```python
from build123d import *

# Parameters (mm, degrees)
SKETCH1_R               = 18
SKETCH1_R_2             = 16
BOSS_EXTRUDE1_DEPTH     = 50
SKETCH3_R               = 18
BOSS_EXTRUDE2_DEPTH     = 2
BOSS_EXTRUDE3_START     = -48
SKETCH3_2_R             = 18
BOSS_EXTRUDE3_DEPTH     = 2
CUT_EXTRUDE1_START      = 14
SKETCH2_W               = 50
SKETCH2_H               = 36
CUT_EXTRUDE1_DEPTH      = 150
CUT_EXTRUDE2_DEPTH      = 57.107040556
CUT_EXTRUDE2_DEPTH_BACK = 57.107040556
SKETCH4_R               = 4


with BuildPart() as part:
    # Sketch1 → Boss-Extrude1 (new body)
    with BuildSketch(Plane.XY):
        Circle(SKETCH1_R)
        Circle(SKETCH1_R_2, mode=Mode.SUBTRACT)
    extrude(amount=BOSS_EXTRUDE1_DEPTH)

    # Sketch3 → Boss-Extrude2 (add)
    with BuildSketch(Plane(origin=(0, 0, 0), x_dir=(-1, 0, 0), z_dir=(0, 0, -1))):
        with Locations(Location((0, 0, 0), (0, 0, 180))):
            Circle(SKETCH3_R)
    extrude(amount=-BOSS_EXTRUDE2_DEPTH)

    # Sketch3<2> → Boss-Extrude3 (add)
    with BuildSketch(Plane(origin=(0, 0, 0), x_dir=(-1, 0, 0), z_dir=(0, 0, -1)).offset(BOSS_EXTRUDE3_START)):
        with Locations(Location((0, 0, 0), (0, 0, 180))):
            Circle(SKETCH3_2_R)
    extrude(amount=-BOSS_EXTRUDE3_DEPTH)

    # Sketch2 → Cut-Extrude1 (cut)
    with BuildSketch(Plane(origin=(0, 0, 0), x_dir=(0, 0, -1), z_dir=(1, 0, 0)).offset(CUT_EXTRUDE1_START)):
        with Locations((-25, 0)):
            Rectangle(SKETCH2_W, SKETCH2_H)
    extrude(amount=CUT_EXTRUDE1_DEPTH, mode=Mode.SUBTRACT)

    # Sketch4 → Cut-Extrude2 (cut, two sides: drawn at the far end of the back side and taken through both)
    with BuildSketch(Plane.XY.offset(50).offset(-CUT_EXTRUDE2_DEPTH_BACK)):
        Circle(SKETCH4_R)
    extrude(amount=CUT_EXTRUDE2_DEPTH + CUT_EXTRUDE2_DEPTH_BACK, mode=Mode.SUBTRACT)


solid = part.part
```
For this review, take the finished solid that the model builds, in its own axes (mm). A direction names the side the tool comes from. Coordinates: 2 decimals unless noted, no trailing zeros. Write each loop counter-clockwise with the first axis right and the second up, starting at its lowest first coordinate (ties: lowest second). Pieces come first, ordered by that corner, then holes. Notation, with made-up numbers: (-18.5, 28) -> (26.5, 28) arc R14 cw to (26.5, 50) -> close; hole circle Ø1 at (18.25, 20). An arc over 180 degrees is marked (long way). Put each result on its own line as item: value.
Q1. Tool access review of faces 4 (the cylindrical face through (-0.867, -3.905, 48.986)), 5 (the flat face through (-5, 0, 2)): name each direction out of +Z, -Z, +X, -X, +Y, -Y from which nothing blocks a thin tool from reaching the whole face with its end or side.
From the geometry:
face 4: +Z, -Z
face 5: none
Q2. Wall thickness on L1, parallel to Z at x = 11.5, y = 3; L2, parallel to Y at x = 0, z = 0.6; L3, parallel to Y at x = 0, z = 25.5: over which ranges is each line inside the solid? List them lowest first.
From the geometry:
L1: z = 0 to 2, 48 to 50
L2: y = -18 to -4, 4 to 18
L3: y = -18 to -16, 16 to 18
Q3. Take a section at B-B, the plane y = 0. State the section outline as (x, z) points.
From the geometry:
outline: (-18, 0) -> (-4, 0) -> (-4, 2) -> (-16, 2) -> (-16, 48) -> (-4, 48) -> (-4, 50) -> (-18, 50) -> close; (4, 0) -> (14, 0) -> (14, 2) -> (4, 2) -> close; (4, 48) -> (14, 48) -> (14, 50) -> (4, 50) -> close
Q4. Take a section at C-C, the plane x = -14.5. State the section outline as (y, z) points.
From the geometry:
outline: (-10.67, 0) -> (10.67, 0) -> (10.67, 50) -> (-10.67, 50) -> close; hole (-6.76, 2) -> (6.76, 2) -> (6.76, 48) -> (-6.76, 48) -> close
Q5. Clearance check with flat-ended pins moving along their axes: pin 1 Ø8 at (x, z) = (-9.5, 34.5) entering from +Y; pin 2 Ø1 at (x, z) = (10, 22.5) entering from +Y; pin 3 Ø13 at (x, y) = (0, 0) entering from +Z; pin 4 Ø1 at (x, z) = (-4, 36) entering from +Y. State where each tip first meets the part, or that it passes through.
From the geometry:
pin 1: stops at y = 17.14
pin 2: stops at y = 15.29
pin 3: stops at z = 50
pin 4: stops at y = 17.66
Q6. Take a section at A-A, the plane x = 0. State the section outline as (y, z) points.
From the geometry:
outline: (-18, 0) -> (-4, 0) -> (-4, 2) -> (-16, 2) -> (-16, 48) -> (-4, 48) -> (-4, 50) -> (-18, 50) -> close; (4, 0) -> (18, 0) -> (18, 50) -> (4, 50) -> (4, 48) -> (16, 48) -> (16, 2) -> (4, 2) -> close
Q7. Take a section at D-D, the plane y = -12. State the section outline as (x, z) points, then the cut area to 3 significant figures.
From the geometry:
outline: (-13.42, 0) -> (13.42, 0) -> (13.42, 50) -> (-13.42, 50) -> close; hole (-10.58, 2) -> (10.58, 2) -> (10.58, 48) -> (-10.58, 48) -> close
area: 368 mm2
Q8. The part is to be moulded in two halves that separate along Y. For faces 1 (the cylindrical face through (-0.867, -3.905, 0.986)), 2 (the cylindrical face through (-17.99, 0.62, 24.65)), 3 (the flat face through (14, 8.4, 25.1)), say which applies: +Y half, -Y half, draft (parallel to the pull), parting line (faces both ways), or undercut.
From the geometry:
face 1: undercut
face 2: parting line
face 3: draft
